Geometry check sheet. Reference: the model listing, model coordinates, mm. Round coordinates to 2 decimals unless told otherwise and drop trailing zeros. Loops run counter-clockwise (first coordinate to the right, second up) from the corner with the lowest first, then second, coordinate; pieces in that order, holes last. Notation, with made-up numbers: (36, 10.25) - (69, 10.25) arc R19 cw to (69, 36.25) - close; hole circle Ø10 at (84, 26.25). An arc over 180 degrees is marked (long way). Answer as CSV lines item,"result". Start each with the question number.
1) Depth check by flat-ended pin: P1, Ø12, axis at x = 44.5, z = -76, coming from the -Y side. Enter the tip coordinate at first touch or a pass-through.
2) Thickness scan on line 1 along X through (y, z) = (2, -89); line 2 along Z through (x, y) = (-169.5, 3). Record the ranges inside material, lowest first.
3) Cross-section at A-A on y = 2. Record the boundary of the cut face in (x, z), and give its area (3 significant figures).
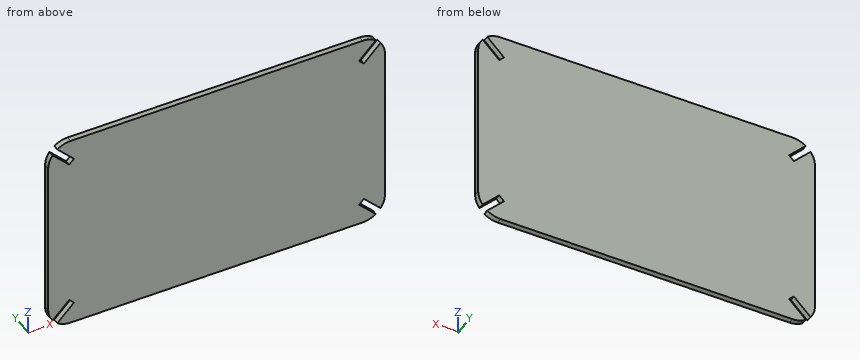
from build123d import *

# Parameters (mm, degrees)
BASE_SUPPORT_DEPTH = 6.35
CUT_EXTRUDE1_DEPTH = 6.35


with BuildPart() as part:
    # Sketch1 → Base Support (new body)
    with BuildSketch(Plane(origin=(0, 0, 0), x_dir=(1, 0, 0), z_dir=(0, 1, 0))):
        with BuildLine():
            Line((-165.1, -114.3), (165.1, -114.3))
            ThreePointArc((165.1, -114.3), (183.060512242, -106.860512242), (190.5, -88.9))
            Line((190.5, -88.9), (190.5, 88.9))
            ThreePointArc((190.5, 88.9), (183.060512242, 106.860512242), (165.1, 114.3))
            Line((165.1, 114.3), (-165.1, 114.3))
            ThreePointArc((-165.1, 114.3), (-183.060512242, 106.860512242), (-190.5, 88.9))
            Line((-190.5, 88.9), (-190.5, -88.9))
            ThreePointArc((-190.5, -88.9), (-183.060512242, -106.860512242), (-165.1, -114.3))
        make_face()
    extrude(amount=BASE_SUPPORT_DEPTH)

    # Sketch2 → Cut-Extrude1 (cut)
    with BuildSketch(Plane(origin=(0, 0, 0), x_dir=(1, 0, 0), z_dir=(0, 1, 0))):
        with BuildLine():
            Line((-180.16323011, -109.351383783), (-161.304692256, -90.492845929))
            Line((-161.304692256, -90.492845929), (-166.692845929, -85.104692256))
            Line((-166.692845929, -85.104692256), (-185.551383783, -103.96323011))
            ThreePointArc((-185.551383783, -103.96323011), (-183.060512242, -106.860512242), (-180.16323011, -109.351383783))
        make_face()
        with BuildLine():
            Line((161.304692256, -90.492845929), (166.692845929, -85.104692256))
            Line((166.692845929, -85.104692256), (185.551383783, -103.96323011))
            ThreePointArc((185.551383783, -103.96323011), (183.060512242, -106.860512242), (180.16323011, -109.351383783))
            Line((180.16323011, -109.351383783), (161.304692256, -90.492845929))
        make_face()
        with BuildLine():
            Line((180.16323011, 109.351383783), (161.304692256, 90.492845929))
            Line((161.304692256, 90.492845929), (166.692845929, 85.104692256))
            Line((166.692845929, 85.104692256), (185.551383783, 103.96323011))
            ThreePointArc((185.551383783, 103.96323011), (183.060512242, 106.860512242), (180.16323011, 109.351383783))
        make_face()
        with BuildLine():
            Line((-166.692845929, 85.104692256), (-185.551383783, 103.96323011))
            ThreePointArc((-185.551383783, 103.96323011), (-183.060512242, 106.860512242), (-180.16323011, 109.351383783))
            Line((-180.16323011, 109.351383783), (-161.304692256, 90.492845929))
            Line((-161.304692256, 90.492845929), (-166.692845929, 85.104692256))
        make_face()
    extrude(amount=CUT_EXTRUDE1_DEPTH, mode=Mode.SUBTRACT)


solid = part.part
Answer block:
1,P1,"stops at y = 0"
2,line 1,"x = -190.5 to -170.59, -162.8 to 162.8, 170.59 to 190.5"
2,line 2,"z = -113.92 to -98.69, -87.91 to 87.91, 98.69 to 113.92"
3,outline,"(-190.5, -88.9) arc R25.4 ccw to (-185.55, -103.96) - (-166.69, -85.1) - (-161.3, -90.49) - (-180.16, -109.35) arc R25.4 ccw to (-165.1, -114.3) - (165.1, -114.3) arc R25.4 ccw to (180.16, -109.35) - (161.3, -90.49) - (166.69, -85.1) - (185.55, -103.96) arc R25.4 ccw to (190.5, -88.9) - (190.5, 88.9) arc R25.4 ccw to (185.55, 103.96) - (166.69, 85.1) - (161.3, 90.49) - (180.16, 109.35) arc R25.4 ccw to (165.1, 114.3) - (-165.1, 114.3) arc R25.4 ccw to (-180.16, 109.35) - (-161.3, 90.49) - (-166.69, 85.1) - (-185.55, 103.96) arc R25.4 ccw to (-190.5, 88.9) - close"
3,area,"85,700 mm^2"
